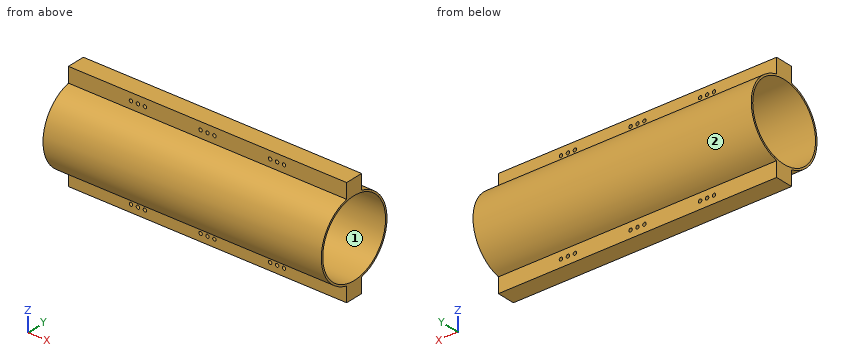
Autodesk Inventor part; units mm, degrees
ref_plane "Work Plane1" through (0, 0, 0) normal (0, 0, 1) x (1, 0, 0)
ref_plane "YZ Plane" through (0, 0, 0) normal (1, 0, 0) x (0, 1, 0)
ref_plane "XZ Plane" through (0, 0, 0) normal (0, 1, 0) x (-1, 0, 0)
sketch "Sketch1" plane through (0, 0, 0) normal (1, 0, 0) x (0, 1, 0)
  circle A0 centre (0, 0) radius 54.5
  circle A1 centre (0, 0) radius 57
  dimension "d0" = 109
  dimension "d1" = 114
extrude "Extrusion1" add sketch "Sketch1" along normal blind 400
sketch "Sketch2" plane through (400, 0, 0) normal (1, 0, 0) x (0, 0, -1)
  circle A0 centre (0, 0) radius 57
  line L0 (-77, 0) -> (-77, 13)
  line L1 (-77, 13) -> (-77, -13)
  line L2 (-77, -13) -> (-55.4977, -13)
  line L3 (-77, 13) -> (-55.4977, 13)
  line L4 (-55.4977, 13) -> (-77, 13)
  line L5 (-77, 13) -> (-77, -13)
  line L6 (-77, -13) -> (-55.4977, -13)
  arc A1 (-55.4977, 13) -> (-55.4977, -13) centre (0, 0) ccw
  dimension "d5" = 13
  dimension "d6" = 26
extrude "Extrusion2" add sketch "Sketch2" against normal blind 400 contours A0 L2 L1 L0 L3
ref_plane "Work Plane1" through (0, 0, 0) normal (0, 0, 1) x (1, 0, 0)
mirror "Mirror1" about plane through (0, 0, 0) normal (0, 0, 1) of "Extrusion2"
sketch "Sketch3" plane through (400, 13, 77) normal (0, 1, 0) x (1, 0, 0)
  line L0 (-400, 21.5023) -> (-400, 0)
  line L1 (0, 0) -> (0, 21.5023)
  circle A0 centre (-200, 10.7511) radius 2.5
  circle A1 centre (-100, 10.7511) radius 2.5
  circle A2 centre (-300, 10.7511) radius 2.5
  circle A3 centre (-190, 10.7511) radius 2.5
  circle A4 centre (-210, 10.7511) radius 2.5
  circle A5 centre (-290, 10.7511) radius 2.5
  circle A6 centre (-310, 10.7511) radius 2.5
  circle A7 centre (-90, 10.7511) radius 2.5
  circle A8 centre (-110, 10.7511) radius 2.5
  point P0 (-400, 77)
extrude "Extrusion4" cut sketch "Sketch3" against normal blind 400
mirror "Mirror3" about plane through (0, 0, 0) normal (0, 0, 1) of "Extrusion4"
Verification items for the finished model (mm, model axes). Face numbers are marked on the shaded views. Give positions to 0.01 mm unless a question says otherwise; leave off trailing zeros. Loops run counter-clockwise (first coordinate to the right, second up) from the corner with the lowest first, then second, coordinate; pieces in that order, holes last. Notation, with made-up numbers: M -37.5,65 L -2.5,65 A26 cw -2.5,98 Z; hole C 88.5,75.5 d9. An arc over 180 degrees is marked long. Return JSON: item names as keys, results as strings.
1) Material ranges on L1, parallel to Z at x = 290, y = 0; L2, parallel to Y at x = 338.5, z = 2.5; L3, parallel to Z at x = 200, y = 4.25, recorded low to high. Write a range as [from, to].
Findings:
{"L1": "z = [-77, -68.75], [-63.75, -54.5], [54.5, 63.75], [68.75, 77]", "L2": "y = [-56.95, -54.44], [54.44, 56.95]", "L3": "z = [-77, -68.75], [-63.75, -54.33], [54.33, 63.75], [68.75, 77]"}
2) Section check C-C, the plane y = -33. Enter the section's corners in (x, z).
Findings:
{"outline": "M 0,-46.48 L 400,-46.48 L 400,-43.37 L 0,-43.37 Z; M 0,43.37 L 400,43.37 L 400,46.48 L 0,46.48 Z"}
3) Section check A-A, the plane y = 0. Count the separate pieces of the cut face and the enclosed holes in it, and give its area (3 significant figures).
Findings:
{"separate pieces": "2", "enclosed holes": "18", "area": "17,600 mm2"}
4) Gauge pin test, flat ends, axial feed: P1, Ø8, axis at x = 200, z = 66.25, coming from the -Y side; P2, Ø1.5, axis at x = 155.5, z = -35.5, coming from the +Y side; P3, Ø10, axis at x = 169.5, z = -25.5, coming from the +Y side. Record the tip position at first contact, or that the pin passes through.
Findings:
{"P1": "stops at y = -13", "P2": "stops at y = 45.18", "P3": "stops at y = 53.19"}
5) Section check D-D, the plane x = 237. Enter the section's corners in (y, z), and give its area (3 significant figures).
Findings:
{"outline": "M -13,-77 L 13,-77 L 13,-55.5 A57 ccw 13,55.5 L 13,77 L -13,77 L -13,55.5 A57 ccw -13,-55.5 Z; hole C 0,0 d109", "area": "1,940 mm2"}
6) Mould release check, pull along Z, two halves, no side actions. Record for the marked faces 1 and 2: released by +Z, released by -Z, zero draft, split by the parting line, or undercut.
Findings:
{"face 1": "undercut", "face 2": "split by the parting line"}
7) Section check B-B, the plane z = -42.5. Enter the section's corners in (x, y).
Findings:
{"outline": "M 0,-37.98 L 400,-37.98 L 400,-34.12 L 0,-34.12 Z; M 0,34.12 L 400,34.12 L 400,37.98 L 0,37.98 Z"}
